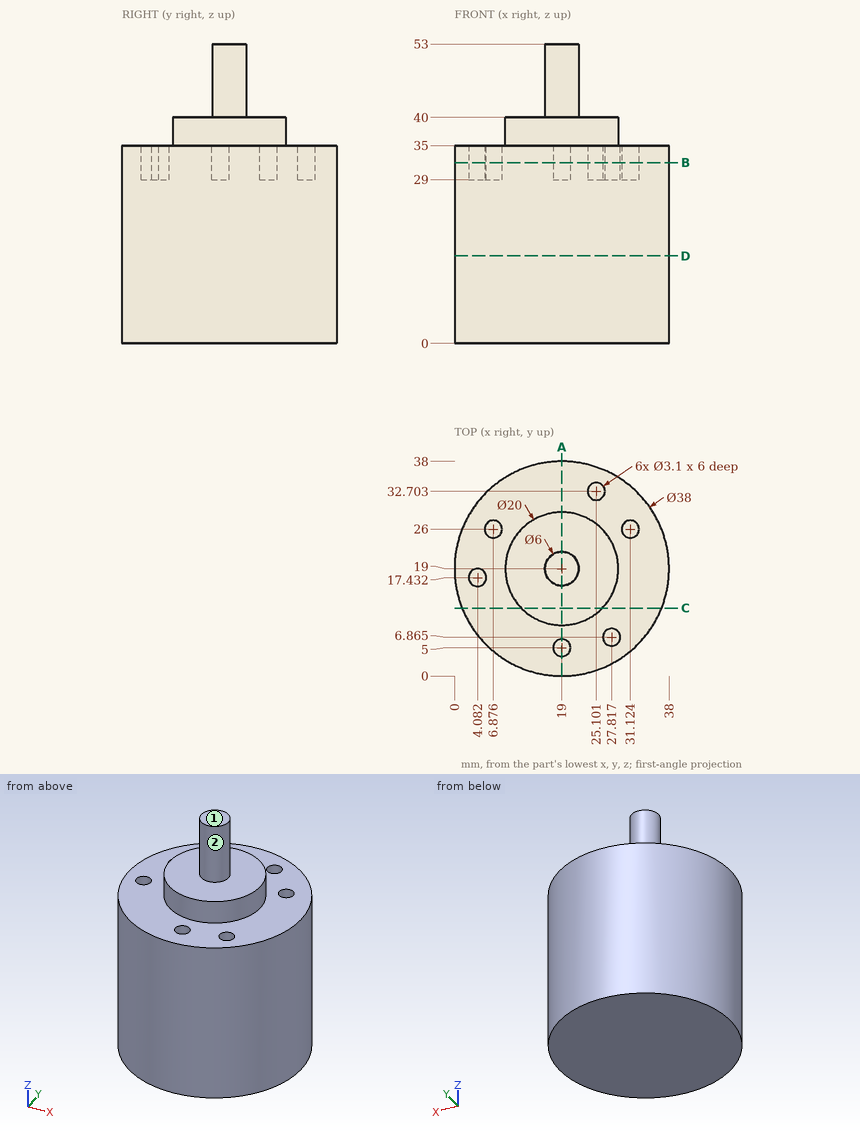
Check sheet for the drawn part. Datum: minimum x, y, z corner. Units: mm. A direction names the side the tool comes from. Round coordinates to 2 decimals unless told otherwise and drop trailing zeros. Order: outer loops, then holes, each group sorted by start corner. A loop starts at its lowest first (then second) coordinate and runs counter-clockwise, first axis right, second up.
(1) Cross-section at A-A, the plane x = 19. Enter the section's corners in (y, z).
(2) Go/stop test with flat-tipped pins: P1, Ø2, axis at x = 31.5, z = 17, coming from the +Y side (1 decimal); P2, Ø12, axis at x = 26, z = 35, coming from the -Y side; P3, Ø2.5, axis at x = 19.5, y = 4.5, coming from the +Z side. Record where each tip stops, or that it passes through.
(3) Cross-section at D-D, the plane z = 15.5. Enter the section's corners in (x, y).
(4) Cross-section at B-B, the plane z = 32. State how many separate pieces and enclosed holes the cut face has, and give its area (3 significant figures).
(5) Cross-section at C-C, the plane y = 12. Enter the section's corners in (x, z).
(6) Access from +Z, -Z, +X, -X, +Y, -Y to the whole of each face (thin tool, end or side, straight path). Record for the marked faces 1 and 2.
(7) Scan lines: probe 1 along X at (y, z) = (26, 31) (1 decimal); probe 2 along Z at (x, y) = (8, 8.5); probe 3 along Z at (x, y) = (17.5, 22). Record each from-to range of solid material in increasing order.
Check sheet entries:
1. outline: (0, 0) - (38, 0) - (38, 35) - (29, 35) - (29, 40) - (22, 40) - (22, 53) - (16, 53) - (16, 40) - (9, 40) - (9, 35) - (6.55, 35) - (6.55, 29) - (3.45, 29) - (3.45, 35) - (0, 35) - close
2. P1: stops at y = 34.1
2. P2: stops at y = 0.03
2. P3: stops at z = 35
3. outline: circle Ø38 at (19, 19)
4. separate pieces: 1
4. enclosed holes: 6
4. area: 1,090 mm2
5. outline: (1.34, 0) - (36.66, 0) - (36.66, 35) - (26.14, 35) - (26.14, 40) - (11.86, 40) - (11.86, 35) - (1.34, 35) - close
6. face 1: +Z, +X, -X, +Y, -Y
6. face 2: +Z
7. probe 1: x = 1.3 to 5.3, 8.4 to 29.6, 32.7 to 36.7
7. probe 2: z = 0 to 35
7. probe 3: z = 0 to 40
